Work out the finished part from the listing and answer in its coordinate system (mm). Coordinates: 2 decimals unless noted, no trailing zeros. Order: outer loops, then holes, each group sorted by start corner. A loop starts at its lowest first (then second) coordinate and runs counter-clockwise, first axis right, second up. Notation, with made-up numbers: (-28, 74) - (-6, 74) arc R21 cw to (-6, 93) - close; hole circle Ø9 at (69.5, 44). An arc over 180 degrees is marked (long way). Answer as a JSON object with one key per item and string values. Group by question number.
1) Each of these flat-tipped pins is pushed along its axis until it touches: P1, Ø1.9, axis at x = 40, y = -40.5, coming from the -Z side; P2, Ø3, axis at x = 42, y = -41.5, coming from the +Z side; P3, Ø3, axis at y = -40.5, z = 139.5, coming from the +X side. Where does it stop, or does it pass through?
2) Find the intervals of material crossed by line 1 along Z through (x, y) = (37.5, -41); line 2 along X through (y, z) = (-39.5, 211.5), in increasing order.
3) Section B-B (z = 218.5) is taken. Give the vertices of the cut face in (x, y).
4) Section A-A (y = -42) is taken. Give the vertices of the cut face in (x, z).
from build123d import *

# Parameters (mm, degrees)
SKETCH1_W           = 76.2
SKETCH1_H           = 6.35
BOSS_EXTRUDE1_DEPTH = 457.2
SKETCH2_W           = 50.8
SKETCH2_H           = 6.35
BOSS_EXTRUDE2_DEPTH = 6.35
SKETCH3_W           = 6.35
SKETCH3_H           = 6.35
CUT_EXTRUDE1_DEPTH  = 6.35
SKETCH4_W           = 6.35
SKETCH4_H           = 6.35
CUT_EXTRUDE2_DEPTH  = 460.399570091


with BuildPart() as part:
    # Sketch1 → Boss-Extrude1 (new body)
    with BuildSketch(Plane.XY):
        with Locations((0, -41.275)):
            Rectangle(SKETCH1_W, SKETCH1_H)
    extrude(amount=BOSS_EXTRUDE1_DEPTH)

    # Sketch2 → Boss-Extrude2 (add)
    with BuildSketch(Plane(origin=(38.1, 0, 0), x_dir=(0, 0, -1), z_dir=(1, 0, 0))):
        with Locations((-381, -41.275)):
            Rectangle(SKETCH2_W, SKETCH2_H)
        with Locations((-279.4, -41.275)):
            Rectangle(SKETCH2_W, SKETCH2_H)
        with Locations((-177.8, -41.275)):
            Rectangle(SKETCH2_W, SKETCH2_H)
        with Locations((-76.2, -41.275)):
            Rectangle(SKETCH2_W, SKETCH2_H)
    extrude(amount=BOSS_EXTRUDE2_DEPTH)

    # Sketch3 → Cut-Extrude1 (cut)
    with BuildSketch(Plane(origin=(0, -38.1, 0), x_dir=(1, 0, 0), z_dir=(0, 1, 0))):
        with Locations((34.925, -107.6625)):
            Rectangle(SKETCH3_W, SKETCH3_H)
    extrude(amount=-CUT_EXTRUDE1_DEPTH, mode=Mode.SUBTRACT)

    # Sketch4 → Cut-Extrude2 (cut, through all)
    with BuildSketch(Plane(origin=(0, -38.1, 0), x_dir=(1, 0, 0), z_dir=(0, 1, 0))):
        with Locations((34.925, -18.7625)):
            Rectangle(SKETCH4_W, SKETCH4_H)
    extrude(amount=-CUT_EXTRUDE2_DEPTH, mode=Mode.SUBTRACT)


solid = part.part
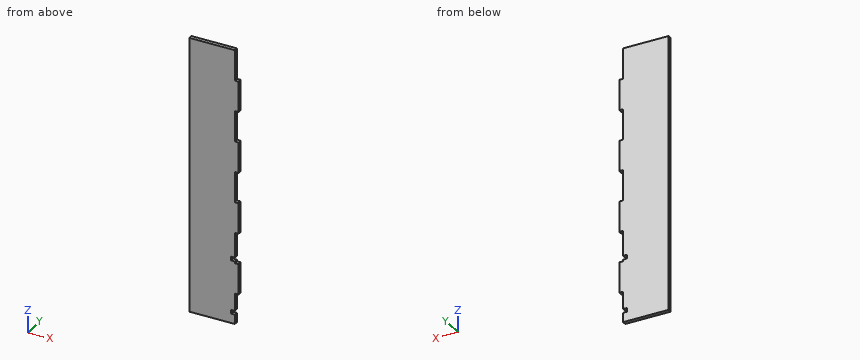
Report:
{
 "1": {"P1": "stops at z = 50.8", "P2": "stops at z = 406.4", "P3": "stops at x = 38.1"},
 "2": {"line 1": "z = 0 to 15.59, 21.94 to 104.49, 110.84 to 457.2", "line 2": "x = -38.1 to 38.1"},
 "3": {"outline": "(-38.1, -44.45) - (38.1, -44.45) - (38.1, -38.1) - (-38.1, -38.1) - close"},
 "4": {"outline": "(-38.1, 0) - (38.1, 0) - (38.1, 15.59) - (31.75, 15.59) - (31.75, 21.94) - (38.1, 21.94) - (38.1, 50.8) - (44.45, 50.8) - (44.45, 101.6) - (38.1, 101.6) - (38.1, 104.49) - (31.75, 104.49) - (31.75, 110.84) - (38.1, 110.84) - (38.1, 152.4) - (44.45, 152.4) - (44.45, 203.2) - (38.1, 203.2) - (38.1, 254) - (44.45, 254) - (44.45, 304.8) - (38.1, 304.8) - (38.1, 355.6) - (44.45, 355.6) - (44.45, 406.4) - (38.1, 406.4) - (38.1, 457.2) - (-38.1, 457.2) - close"}
}
